from build123d import *

# Parameters (mm, degrees)
SKETCH1_W                    = 1343.025
SKETCH1_H                    = 527.05
BOSS_EXTRUDE1_DEPTH          = 17.78
FILLET1_R                    = 6.35
F_1_8_0_125_DIAMETER_HOLE1_D = 3.175
SKETCH5_W                    = 152.4
SKETCH5_H                    = 400.05
CUT_EXTRUDE1_DEPTH           = 18.78
FILLET2_R                    = 6.35


with BuildPart() as part:
    # Sketch1 → Boss-Extrude1 (new body)
    with BuildSketch(Plane(origin=(0, 0, 0), x_dir=(1, 0, 0), z_dir=(0, 1, 0))):
        Rectangle(SKETCH1_W, SKETCH1_H)
    extrude(amount=BOSS_EXTRUDE1_DEPTH)

    # Fillet1
    fillet1_edges = [part.edges().sort_by_distance(p)[0] for p in [
        (671.5125, 8.89, 263.525),
        (-671.5125, 8.89, 263.525),
        (-671.5125, 8.89, -263.525),
        (671.5125, 8.89, -263.525),
    ]]
    fillet(fillet1_edges, radius=FILLET1_R)

    # 1/8 (0.125) Diameter Hole1 (through all)
    with Locations(Plane(origin=(0, 17.78, 0), x_dir=(1, 0, 0), z_dir=(0, 1, 0))):
        with Locations((0, 0), (457.2, 152.4), (-457.2, -152.4), (-457.2, 152.4), (457.2, -152.4)):
            Hole(F_1_8_0_125_DIAMETER_HOLE1_D / 2)

    # Sketch5 → Cut-Extrude1 (cut, through all)
    with BuildSketch(Plane(origin=(0, 17.78, 0), x_dir=(1, 0, 0), z_dir=(0, 1, 0))):
        Polygon((-406.4, 200.025), (406.4, 200.025), (0, 38.1), align=None)
        Polygon((0, -38.1), (-406.4, -200.025), (406.4, -200.025), align=None)
        Polygon((406.4, 146.74453125), (406.4, -146.74453125), (38.1, 0), align=None)
        Polygon((-406.4, 146.74453125), (-38.1, 0), (-406.4, -146.74453125), align=None)
        with Locations((550.8625, 0)):
            Rectangle(SKETCH5_W, SKETCH5_H)
        with Locations((-550.8625, 0)):
            Rectangle(SKETCH5_W, SKETCH5_H)
    extrude(amount=-CUT_EXTRUDE1_DEPTH, mode=Mode.SUBTRACT)

    # Fillet2
    fillet2_edges = [part.edges().sort_by_distance(p)[0] for p in [
        (-474.6625, 8.89, -200.025),
        (-474.6625, 8.89, 200.025),
        (-627.0625, 8.89, 200.025),
        (-627.0625, 8.89, -200.025),
        (-406.4, 8.89, 146.74453125),
        (-406.4, 8.89, -146.74453125),
        (-38.1, 8.89, 0),
        (627.0625, 8.89, -200.025),
        (627.0625, 8.89, 200.025),
        (474.6625, 8.89, 200.025),
        (474.6625, 8.89, -200.025),
        (0, 8.89, 38.1),
        (406.4, 8.89, 200.025),
        (-406.4, 8.89, 200.025),
        (38.1, 8.89, 0),
        (406.4, 8.89, -146.74453125),
        (406.4, 8.89, 146.74453125),
        (406.4, 8.89, -200.025),
        (0, 8.89, -38.1),
        (-406.4, 8.89, -200.025),
    ]]
    fillet(fillet2_edges, radius=FILLET2_R)


solid = part.part
Work out the finished part from the listing and answer in its coordinate system (mm). A direction names the side the tool comes from. Coordinates: 2 decimals unless noted, no trailing zeros. Write each loop counter-clockwise with the first axis right and the second up, starting at its lowest first coordinate (ties: lowest second). Pieces come first, ordered by that corner, then holes. Notation, with made-up numbers: M 2,74.25 L 30,74.25 A8 ccw 30,87.25 Z; hole C 71.25,38 d4. An arc over 180 degrees is marked long. Write item = value, one per line.
1. Flat-ended cylindrical pins translate along their axes: pin 1 (3 mm diameter, centred on x = -457.2, z = 152.4, fed in from -Y); pin 2 (3.5 mm diameter, centred on x = 0, z = 0, fed in from -Y). Find the tip coordinate at first contact, or state that the pin passes through.
Solution:
pin_1 = through
pin_2 = 0
2. Determine the mould class of faces 1 (the face through (-186.391, 9.014, 112.365)), 2 (the face through (-9, 0, -4)) for opening direction X: released by +X, released by -X, zero draft, split by the parting line, or undercut.
Solution:
face_1 = undercut
face_2 = zero draft
3. The part is cut by section B-B (x = -283). Determine the outline of the cut face in (y, z) (3 decimals).
Solution:
outline = M 0,-263.525 L 17.78,-263.525 L 17.78,-200.025 L 0,-200.025 Z; M 0,-150.858 L 17.78,-150.858 L 17.78,-97.577 L 0,-97.577 Z; M 0,97.577 L 17.78,97.577 L 17.78,150.858 L 0,150.858 Z; M 0,200.025 L 17.78,200.025 L 17.78,263.525 L 0,263.525 Z
4. Straight lines are drawn through the part: line 1 (Z direction, x = -457.2, y = 9) (1 decimal); line 2 (Z direction, x = 400, y = 3) (3 decimals); line 3 (Z direction, x = -534.5, y = 8.5) (3 decimals). For each, find the intervals that lie inside material, in ascending order. Write a range as from..to.
Solution:
line_1 = -263.5..-154, -150.8..150.8, 154..263.5
line_2 = -263.525..-143.729, 143.729..263.525
line_3 = -263.525..-200.025, 200.025..263.525
5. The part is cut by section A-A (z = -87). Determine the outline of the cut face in (x, y), then the cut area to 3 significant figures.
Solution:
outline = M -671.51,0 L -627.06,0 L -627.06,17.78 L -671.51,17.78 Z; M -474.66,0 L -406.4,0 L -406.4,17.78 L -474.66,17.78 Z; M -256.45,0 L -122.73,0 L -122.73,17.78 L -256.45,17.78 Z; M 122.73,0 L 256.45,0 L 256.45,17.78 L 122.73,17.78 Z; M 406.4,0 L 474.66,0 L 474.66,17.78 L 406.4,17.78 Z; M 627.06,0 L 671.51,0 L 671.51,17.78 L 627.06,17.78 Z
area = 8,760 mm2
6. The part is cut by section C-C (y = 11.75). State how many separate pieces and enclosed holes the cut face has, then the cut area to 3 significant figures.
Solution:
separate_pieces = 1
enclosed_holes = 11
area = 347,000 mm2
7. For faces 3 (the face through (-9, 17.78, -4)), 4 (the face through (227.72, 9.01, 75.55)), determine the directions among +Z, -Z, +X, -X, +Y, -Y from which every point of the face is accessible in a straight line to the end or side of a thin tool.
Solution:
face_3 = +Z, -Z, +X, -X, +Y
face_4 = +Y, -Y
